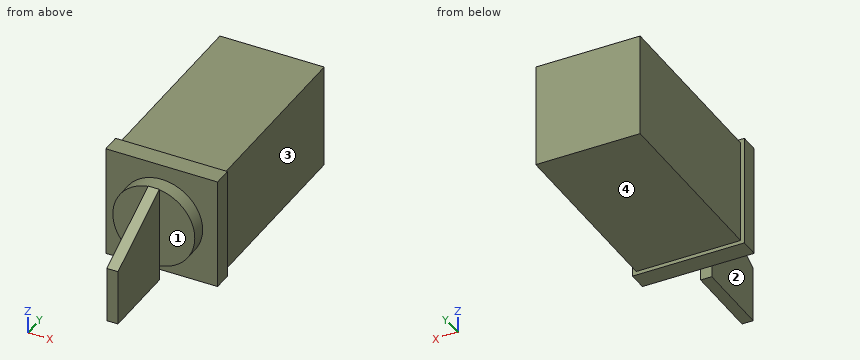
from build123d import *

# Parameters (mm, degrees)
F0_W     = 28
F0_H     = 28
F1_DEPTH = 51
F2_W     = 30
F2_H     = 30
F3_DEPTH = 5
F4_R     = 11
F5_DEPTH = 4
F6_W     = 3
F6_H     = 15
F7_DEPTH = 21
F9_DEPTH = 3


with BuildPart() as f1:
    # F0 (on Front) → F1 (new body)
    with BuildSketch(Plane.XZ):
        Rectangle(F0_W, F0_H)
    extrude(amount=-F1_DEPTH)

    # F2 (on Front) → F3 (join)
    with BuildSketch(Plane.XZ):
        Rectangle(F2_W, F2_H)
    extrude(amount=F3_DEPTH)

    # F4 (on face) → F5 (join)
    with BuildSketch(Plane.XZ.offset(5)):
        Circle(F4_R)
    extrude(amount=F5_DEPTH)

    # F6 (on face) → F7 (join)
    with BuildSketch(Plane.XZ.offset(9)):
        with Locations((0, -7.5)):
            Rectangle(F6_W, F6_H)
    extrude(amount=F7_DEPTH)

    # F8 (on face) → F9 (join)
    with BuildSketch(Plane.YZ.offset(1.5)):
        Polygon((-9, 11), (-30, 0), (-9, 0), align=None)
    extrude(amount=-F9_DEPTH)


solid = f1.part
Can you work these out from the model? Positions are in its coordinate system, mm. Face numbers are marked on the shaded views. A direction names the side the tool comes from. Give positions to 0.01 mm unless a question says otherwise; leave off trailing zeros. Loops run counter-clockwise (first coordinate to the right, second up) from the corner with the lowest first, then second, coordinate; pieces in that order, holes last. Notation, with made-up numbers: (49, 20) -> (99, 20) arc R34 ccw to (99, 58) -> close; hole circle Ø10 at (29, 0.5). An arc over 180 degrees is marked (long way). Return JSON: item names as keys, results as strings.
Q1. For pin 1 Ø9 at (x, z) = (0.5, 2) entering from -Y; pin 2 Ø5 at (x, y) = (-0.5, 32.5) entering from +Z; pin 3 Ø5 at (y, z) = (39.5, 4) entering from -X; pin 4 Ø1.5 at (x, z) = (5.5, 2) entering from -Y, each with a flat end and sliding along its axis, tell me the tip position at first contact or that it passes through.
Checks:
{"pin 1": "stops at y = -30", "pin 2": "stops at z = 14", "pin 3": "stops at x = -14", "pin 4": "stops at y = -9"}
Q2. I need wall thicknesses on probe 1 along X at (y, z) = (10, -10); probe 2 along Y at (x, z) = (6.5, 12.5). Which ranges of each line are inside material? Lowest first, please.
Checks:
{"probe 1": "x = -14 to 14", "probe 2": "y = -5 to 51"}
Q3. I want a section at A-A, the plane z = 12.25. List the corners of the cut face in (x, y) for me, then the cut area to 3 significant figures.
Checks:
{"outline": "(-15, -5) -> (15, -5) -> (15, 0) -> (14, 0) -> (14, 51) -> (-14, 51) -> (-14, 0) -> (-15, 0) -> close", "area": "1,580 mm2"}
Q4. I want a section at D-D, the plane z = 6. List the corners of the cut face in (x, y) for me.
Checks:
{"outline": "(-15, -5) -> (-9.22, -5) -> (-9.22, -9) -> (-1.5, -9) -> (-1.5, -18.55) -> (1.5, -18.55) -> (1.5, -9) -> (9.22, -9) -> (9.22, -5) -> (15, -5) -> (15, 0) -> (14, 0) -> (14, 51) -> (-14, 51) -> (-14, 0) -> (-15, 0) -> close"}
Q5. I want a section at C-C, the plane y = 39.5. List the corners of the cut face in (x, z) for me, then the cut area to 3 significant figures.
Checks:
{"outline": "(-14, -14) -> (14, -14) -> (14, 14) -> (-14, 14) -> close", "area": "784 mm2"}
Q6. I want a section at B-B, the plane x = 2.25. List the corners of the cut face in (y, z) for me.
Checks:
{"outline": "(-9, -10.77) -> (-5, -10.77) -> (-5, -15) -> (0, -15) -> (0, -14) -> (51, -14) -> (51, 14) -> (0, 14) -> (0, 15) -> (-5, 15) -> (-5, 10.77) -> (-9, 10.77) -> close"}
Q7. On a 3-axis mill with a long thin cutter (end or side, diameter ignored), from which of +Z, -Z, +X, -X, +Y, -Y can I reach the whole of each face in a straight line? I mean the marked faces 1, 2, 3 and 4. Say none if no direction works.
Checks:
{"face 1": "+Z, -Z, +X, -Y", "face 2": "+Z, -Z, -X, -Y", "face 3": "+Z, -Z, +X, +Y", "face 4": "-Z, +X, -X, +Y"}
